Model file for the job. Use its own axes, mm. Give positions to 0.01 mm unless a question says otherwise; leave off trailing zeros. Write each loop counter-clockwise with the first axis right and the second up, starting at its lowest first coordinate (ties: lowest second). Pieces come first, ordered by that corner, then holes. Notation, with made-up numbers: (26.5, 24.5) - (81.5, 24.5) arc R33 ccw to (81.5, 52.5) - close; hole circle Ø2 at (86, 32). An arc over 180 degrees is marked (long way). Use CSV: the item, a comma, the result in double quotes.
from build123d import *

# Parameters (mm, degrees)
SKETCH1_R           = 2.5
BOSS_EXTRUDE1_DEPTH = 2.5


with BuildPart() as part:
    # Sketch1 → Boss-Extrude1 (new body)
    with BuildSketch(Plane.XY.offset(1.25)):
        Polygon((-12.7, 37.846), (-12.7, -37.846), (-6.35, -44.196), (6.35, -44.196), (12.7, -37.846), (12.7, 37.846), (6.35, 44.196), (-6.35, 44.196), align=None)
        with Locations((0, -38.1)):
            Circle(SKETCH1_R, mode=Mode.SUBTRACT)
        with Locations((0, -25.4)):
            Circle(SKETCH1_R, mode=Mode.SUBTRACT)
        with Locations((0, -12.7)):
            Circle(SKETCH1_R, mode=Mode.SUBTRACT)
        Circle(SKETCH1_R, mode=Mode.SUBTRACT)
        with Locations((0, 12.7)):
            Circle(SKETCH1_R, mode=Mode.SUBTRACT)
        with Locations((0, 38.1)):
            Circle(SKETCH1_R, mode=Mode.SUBTRACT)
        with Locations((0, 25.4)):
            Circle(SKETCH1_R, mode=Mode.SUBTRACT)
    extrude(amount=-BOSS_EXTRUDE1_DEPTH)


solid = part.part
(1) Flat gauge pin, fed straight in: P1, Ø4, axis at x = 0, y = -12.7, coming from the +Z side. Where does the tip first touch, or does it go through?
Checked values:
P1,"passes through"
(2) Saw through at D-D, the plane x = -10.5. List the corners of the cut face in (y, z), then the cut area to 3 significant figures.
Checked values:
outline,"(-40.05, -1.25) - (40.05, -1.25) - (40.05, 1.25) - (-40.05, 1.25) - close"
area,"200 mm^2"
(3) Saw through at A-A, the plane y = -25.4. List the corners of the cut face in (x, z).
Checked values:
outline,"(-12.7, -1.25) - (-2.5, -1.25) - (-2.5, 1.25) - (-12.7, 1.25) - close; (2.5, -1.25) - (12.7, -1.25) - (12.7, 1.25) - (2.5, 1.25) - close"
(4) Saw through at C-C, the plane z = 0.6. List the corners of the cut face in (x, y), then the cut area to 3 significant figures.
Checked values:
outline,"(-12.7, -37.85) - (-6.35, -44.2) - (6.35, -44.2) - (12.7, -37.85) - (12.7, 37.85) - (6.35, 44.2) - (-6.35, 44.2) - (-12.7, 37.85) - close; hole circle Ø5 at (0, -38.1); hole circle Ø5 at (0, -25.4); hole circle Ø5 at (0, -12.7); hole circle Ø5 at (0, 0); hole circle Ø5 at (0, 12.7); hole circle Ø5 at (0, 25.4); hole circle Ø5 at (0, 38.1)"
area,"2,030 mm^2"
(5) Wall check: probe 1 along X at (y, z) = (-15, -0.9); probe 2 along X at (y, z) = (1, -0.6); probe 3 along Y at (x, z) = (-7.75, -0.5). Give the ranges that are in metal, low to high. Write a range as [from, to].
Checked values:
probe 1,"x = [-12.7, -0.98], [0.98, 12.7]"
probe 2,"x = [-12.7, -2.29], [2.29, 12.7]"
probe 3,"y = [-42.8, 42.8]"
(6) Saw through at B-B, the plane x = -1.5. Count the separate pieces of the cut face and the enclosed holes in it, then the cut area to 3 significant figures.
Checked values:
separate pieces,"8"
enclosed holes,"0"
area,"151 mm^2"
(7) Pull direction X, two halves, no side cores. Call faces 1 (the face through (3, 1, 1.25)), 2 (the face through (12.7, -1, 0)), 3 (the face through (-0.33, 27.88, 0.02)): released by +X, released by -X, zero draft, split by the parting line, or undercut.
Checked values:
face 1,"zero draft"
face 2,"released by +X"
face 3,"undercut"
